```python
from build123d import *

# Parameters (mm, degrees)
CROQUIS1_W              = 40
CROQUIS1_H              = 15
SALIENTE_EXTRUIR1_DEPTH = 5
CROQUIS2_W              = 5
CROQUIS2_H              = 15
SALIENTE_EXTRUIR2_DEPTH = 20
CROQUIS3_R              = 4.25
CORTAR_EXTRUIR1_DEPTH   = 20
CORTAR_EXTRUIR2_DEPTH   = 20


with BuildPart() as part:
    # Croquis1 → Saliente-Extruir1 (new body)
    with BuildSketch(Plane(origin=(0, 0, 0), x_dir=(1, 0, 0), z_dir=(0, 1, 0))):
        Rectangle(CROQUIS1_W, CROQUIS1_H)
    extrude(amount=SALIENTE_EXTRUIR1_DEPTH)

    # Croquis2 → Saliente-Extruir2 (add)
    with BuildSketch(Plane(origin=(0, 5, 0), x_dir=(1, 0, 0), z_dir=(0, 1, 0))):
        with Locations((17.5, 0)):
            Rectangle(CROQUIS2_W, CROQUIS2_H)
    extrude(amount=SALIENTE_EXTRUIR2_DEPTH)

    # Croquis3 → Cortar-Extruir1 (cut)
    with BuildSketch(Plane(origin=(20, 0, 0), x_dir=(0, 0, -1), z_dir=(1, 0, 0))):
        with Locations((0, 15)):
            Circle(CROQUIS3_R)
    extrude(amount=-CORTAR_EXTRUIR1_DEPTH, mode=Mode.SUBTRACT)

    # Croquis4 → Cortar-Extruir2 (cut)
    with BuildSketch(Plane(origin=(0, 5, 0), x_dir=(1, 0, 0), z_dir=(0, 1, 0))):
        with BuildLine():
            Line((-16.5, 2), (-7, 2))
            ThreePointArc((-7, 2), (-5, 0), (-7, -2))
            Line((-7, -2), (-16.5, -2))
            ThreePointArc((-16.5, -2), (-18.5, 0), (-16.5, 2))
        make_face()
        with BuildLine():
            Line((11.5, -2), (2, -2))
            ThreePointArc((2, -2), (0, 0), (2, 2))
            Line((2, 2), (11.5, 2))
            ThreePointArc((11.5, 2), (13.5, 0), (11.5, -2))
        make_face()
    extrude(amount=-CORTAR_EXTRUIR2_DEPTH, mode=Mode.SUBTRACT)


solid = part.part
```
Can you work these out from the model? Positions are in its coordinate system, mm. A direction names the side the tool comes from. Give positions to 0.01 mm unless a question says otherwise; leave off trailing zeros. Write each loop counter-clockwise with the first axis right and the second up, starting at its lowest first coordinate (ties: lowest second). Pieces come first, ordered by that corner, then holes. Notation, with made-up numbers: (-4.75, 89) - (18.25, 89) arc R8 ccw to (18.25, 98) - close; hole circle Ø10 at (14, -5.5). An arc over 180 degrees is marked (long way). Write item = value, one per line. Start each with the question number.
1. Imagine slicing it at B-B (x = -14.5). Please give me the cut outline in (y, z).
2. Imagine slicing it at D-D (y = 1.75). Please give me the cut outline in (x, z).
3. Imagine slicing it at A-A (y = 15). Please give me the cut outline in (x, z).
4. Please list where these lines run through material, in increasing order: line 1 (Z direction, x = 9, y = 3.5); line 2 (Y direction, x = 17.5, z = 0); line 3 (X direction, y = 20.25, z = -3).
5. On a 3-axis mill with a long thin cutter (end or side, diameter ignored), from which of +Z, -Z, +X, -X, +Y, -Y can I reach the whole of each face in a straight line? I mean faces 1 (the face through (15, 10, 0)), 2 (the face through (17, 25, 0)), 3 (the face through (-5, 3, 0)). Say none if no direction works.
6. For pin 1 (7.5 mm diameter, centred on x = 0.5, z = 3, fed in from +Y); pin 2 (7.5 mm diameter, centred on y = 14, z = -2, fed in from -X); pin 3 (7 mm diameter, centred on y = 15, z = 0, fed in from +X), each with a flat end and sliding along its axis, tell me the tip position at first contact or that it passes through.
7. Imagine slicing it at C-C (z = -0.75). Please give me the cut outline in (x, y).
8. Thinking about a two-plate mould opening in Z: for faces 4 (the face through (6, 4, -7.5)), 5 (the face through (17.54, 10.85, 0.92)), 6 (the face through (-0.3, 0, -0.1)), which applies, released by +Z, released by -Z, zero draft, split by the parting line, or undercut?
Worked answers:
q1.outline = (0, -7.5) - (5, -7.5) - (5, -2) - (0, -2) - close; (0, 2) - (5, 2) - (5, 7.5) - (0, 7.5) - close
q2.outline = (-20, -7.5) - (20, -7.5) - (20, 7.5) - (-20, 7.5) - close; hole (-16.5, -2) - (-7, -2) arc R2 ccw to (-7, 2) - (-16.5, 2) arc R2 ccw to start; hole (2, -2) - (11.5, -2) arc R2 ccw to (11.5, 2) - (2, 2) arc R2 ccw to start
q3.outline = (15, -7.5) - (20, -7.5) - (20, -4.25) - (15, -4.25) - close; (15, 4.25) - (20, 4.25) - (20, 7.5) - (15, 7.5) - close
q4.line_1 = -7.5 to -2, 2 to 7.5
q4.line_2 = 0 to 10.75, 19.25 to 25
q4.line_3 = 15 to 20
q5.face_1 = +Z, -Z, -X, +Y
q5.face_2 = +Z, -Z, +X, -X, +Y
q5.face_3 = +Y, -Y
q6.pin_1 = 5
q6.pin_2 = 15
q6.pin_3 = through
q7.outline = (-20, 0) - (-18.35, 0) - (-18.35, 5) - (-20, 5) - close; (-5.15, 0) - (0.15, 0) - (0.15, 5) - (-5.15, 5) - close; (13.35, 0) - (20, 0) - (20, 10.82) - (15, 10.82) - (15, 5) - (13.35, 5) - close; (15, 19.18) - (20, 19.18) - (20, 25) - (15, 25) - close
q8.face_4 = released by -Z
q8.face_5 = undercut
q8.face_6 = zero draft
